Drawing for the job (mm, zero at the part's lowest x, y, z). A direction names the side the tool comes from. Give positions to 0.01 mm unless a question says otherwise; leave off trailing zeros. Loops run counter-clockwise (first coordinate to the right, second up) from the corner with the lowest first, then second, coordinate; pieces in that order, holes last. Notation, with made-up numbers: (34.25, 51.25) -> (77.25, 51.25) arc R12 ccw to (77.25, 71.25) -> close; hole circle Ø11 at (6, 30). An arc over 180 degrees is marked (long way). Use CSV: the item, a comma, the result in double quotes. Start each with the question number.
(1) Cut at A-A on z = 13. Write the cut outline in (x, y), then the cut area to 3 significant figures.
(2) Cut at C-C on y = 13.25. Write the cut outline in (x, z), then the cut area to 3 significant figures.
(3) Flat gauge pins, fed straight in: pin 1 (5 mm diameter, centred on x = 97, y = 16, fed in from -Z); pin 2 (4 mm diameter, centred on x = 87.5, z = 21.5, fed in from +Y); pin 3 (1 mm diameter, centred on y = 11, z = 7.5, fed in from -X); pin 4 (1.5 mm diameter, centred on x = 97.5, y = 3.5, fed in from +Z). Where does each tip first touch, or does it go through?
(4) Cut at B-B on x = 35. Write the cut outline in (y, z), then the cut area to 3 significant figures.
(5) Drill centre lines: probe 1 along Z at (x, y) = (27.5, 10); probe 2 along X at (y, z) = (7.5, 24); probe 3 along Y at (x, z) = (46.5, 25.5). Where is each one in solid material? Low to high.
(6) 3-axis set-ups, long thin cutter, end or side, ignore diameter. For the marked faces 1, 2 and 3: which of +Z, -Z, +X, -X, +Y, -Y reach the whole face in a straight line?
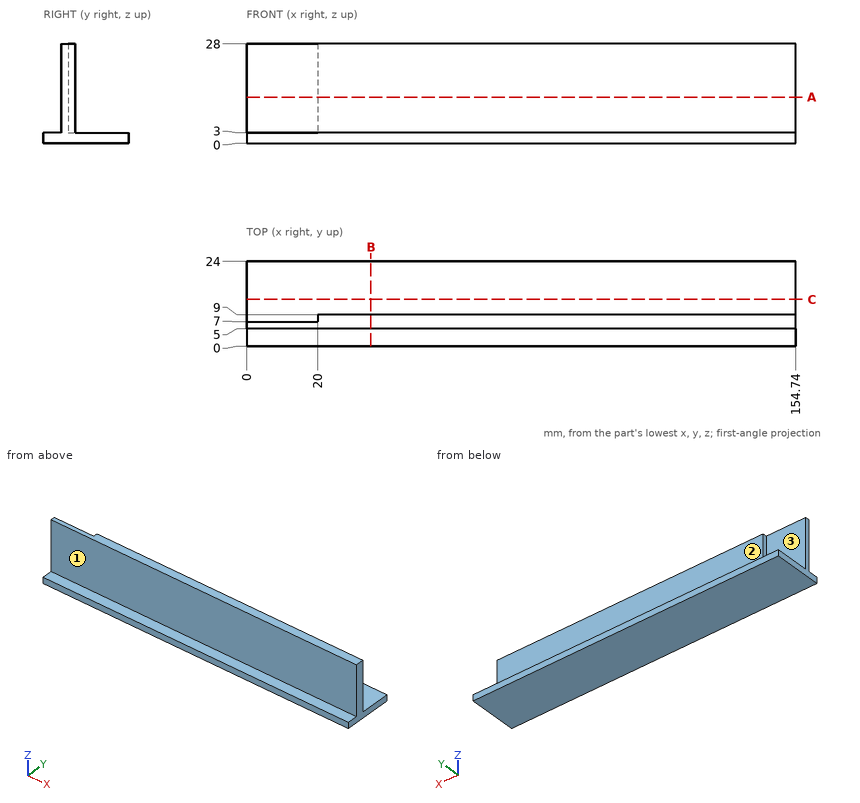
Check result:
1,outline,"(0, 5) -> (154.74, 5) -> (154.74, 9) -> (20, 9) -> (20, 7) -> (0, 7) -> close"
1,area,"579 mm²"
2,outline,"(0, 0) -> (154.74, 0) -> (154.74, 3) -> (0, 3) -> close"
2,area,"464 mm²"
3,pin 1,"z = 0"
3,pin 2,"y = 9"
3,pin 3,"through"
3,pin 4,"z = 3"
4,outline,"(0, 0) -> (24, 0) -> (24, 3) -> (9, 3) -> (9, 28) -> (5, 28) -> (5, 3) -> (0, 3) -> close"
4,area,"172 mm²"
5,probe 1,"0 to 3"
5,probe 2,"20 to 154.74"
5,probe 3,"5 to 9"
6,face 1,"+Z, +X, -X, -Y"
6,face 2,"+Z, +X, -X, +Y"
6,face 3,"+Z, -X, +Y"
